from build123d import *

# Parameters (mm, degrees)
EXTRUDE_1_DEPTH     = 5
SKETCH_1_3_W        = 20
SKETCH_1_3_H        = 5
EXTRUDE_2_DEPTH     = 10
SKETCH_1_4_W        = 20
SKETCH_1_4_H        = 5
EXTRUDE_3_DEPTH     = 25
SKETCH_2_R          = 2.5
CUT_EXTRUDE_1_DEPTH = 25
CUT_EXTRUDE_2_DEPTH = 5
SKETCH_4_R          = 2.5
EXTRUDE_4_DEPTH     = 5


with BuildPart() as part:
    # 草圖1 → 填料-伸長1 (new body)
    with BuildSketch(Plane(origin=(0, 0, 0), x_dir=(1, 0, 0), z_dir=(0, 1, 0))):
        with BuildLine():
            Line((20, 10), (20, 5))
            Line((20, 5), (20, 0))
            ThreePointArc((20, 0), (23.535533906, 1.464466094), (25, 5))
            Line((25, 5), (25, 10))
            Line((25, 10), (20, 10))
        make_face()
    extrude(amount=EXTRUDE_1_DEPTH)

    # 草圖1<3> → 填料-伸長2 (add)
    with BuildSketch(Plane(origin=(0, 0, 0), x_dir=(1, 0, 0), z_dir=(0, 1, 0))):
        with Locations((10, 2.5)):
            Rectangle(SKETCH_1_3_W, SKETCH_1_3_H)
    extrude(amount=EXTRUDE_2_DEPTH)

    # 草圖1<4> → 填料-伸長3 (add)
    with BuildSketch(Plane(origin=(0, 0, 0), x_dir=(1, 0, 0), z_dir=(0, 1, 0))):
        with Locations((10, 7.5)):
            Rectangle(SKETCH_1_4_W, SKETCH_1_4_H)
    extrude(amount=EXTRUDE_3_DEPTH)

    # 草圖2 → 除料-伸長1 (cut)
    with BuildSketch(Plane.XY.offset(-5)):
        with Locations((15, 15)):
            Circle(SKETCH_2_R)
        Polygon((10, 25), (20, 20), (20, 25), align=None)
    extrude(amount=-CUT_EXTRUDE_1_DEPTH, mode=Mode.SUBTRACT)

    # 草圖3 → 除料-伸長2 (cut)
    with BuildSketch(Plane.XY):
        Polygon((20, 5), (5, 10), (20, 10), align=None)
    extrude(amount=-CUT_EXTRUDE_2_DEPTH, mode=Mode.SUBTRACT)

    # 草圖4 → 填料-伸長4 (add)
    with BuildSketch(Plane(origin=(0, 0, 0), x_dir=(0, 0, -1), z_dir=(1, 0, 0))):
        with BuildLine():
            Line((0, 10), (-10, 10))
            ThreePointArc((-10, 10), (-13.535533906, 8.535533906), (-15, 5))
            Line((-15, 5), (-15, 0))
            Line((-15, 0), (0, 0))
            Line((0, 0), (0, 10))
        make_face()
        with Locations((-10, 5)):
            Circle(SKETCH_4_R, mode=Mode.SUBTRACT)
    extrude(amount=EXTRUDE_4_DEPTH)


solid = part.part
Could you check a few things on this model? Use its own coordinates, in mm. A direction names the side the tool comes from. Give positions to 0.01 mm unless a question says otherwise; leave off trailing zeros. Order: outer loops, then holes, each group sorted by start corner. A loop starts at its lowest first (then second) coordinate and runs counter-clockwise, first axis right, second up.
1. Suppose I cut it at C-C (x = 11). List the corners of the cut face in (y, z) for me.
2. Suppose I cut it at A-A (y = 13.5). List the corners of the cut face in (x, z) for me, plus the area to 3 significant figures.
3. I need wall thicknesses on L1, parallel to Z at x = 4.5, y = 10.5; L2, parallel to Y at x = 15, z = -8.4; L3, parallel to X at y = 7.5, z = 7.75. Which ranges of each line are inside material? Lowest first, please.
4. We'd pull the mould along Z, two halves only. Please class faces 4 (the cylindrical face through (2.46, 6.69, 11.84)), 5 (the flat face through (25, 2, -7)), 6 (the flat face through (12, 4, 0)): pulls with the +Z half, pulls with the -Z half, needs draft (parallel to the pull), parting line crosses it, or undercut.
5. For faces 1 (the flat face through (12.605, 7.465, -2.465)), 2 (the flat face through (22, 5, -5)), 3 (the flat face through (5, 5, 6)), which set-ups out of +Z, -Z, +X, -X, +Y, -Y let a thin tool reach every point of the face, with its end or its side?
6. Suppose I cut it at D-D (z = -1). List the corners of the cut face in (x, y) for me, plus the area to 4 significant figures.
7. Suppose I cut it at B-B (x = 2.5). List the corners of the cut face in (y, z) for me, plus the area to 3 significant figures.
8. Will these pins go through, and if not, where does the flat tip stop? P1, Ø8, axis at y = 6, z = 5.5, coming from the +X side; P2, Ø10, axis at x = 8, y = 19, coming from the +Z side; P3, Ø4, axis at x = 2, z = 0.5, coming from the +Y side.
Solved:
1. outline: (0, -10) - (24.5, -10) - (24.5, -5) - (8, -5) - (8, 0) - (0, 0) - close
2. outline: (0, -10) - (13, -10) - (13, -5) - (0, -5) - close; (17, -10) - (20, -10) - (20, -5) - (17, -5) - close
2. area: 80.0 mm2
3. L1: z = -10 to -5
3. L2: y = 0 to 12.5, 17.5 to 22.5
3. L3: x = 0 to 5
4. face 4: undercut
4. face 5: needs draft
4. face 6: pulls with the +Z half
5. face 1: +Z, +X, +Y
5. face 2: +Z, -Z, +X, +Y
5. face 3: +Z, +X, +Y, -Y
6. outline: (0, 0) - (23, 0) - (23, 5) - (20, 5) - (5, 10) - (0, 10) - close
6. area: 177.5 mm2
7. outline: (0, -10) - (25, -10) - (25, -5) - (10, -5) - (10, 10) arc R5 ccw to (5, 15) - (0, 15) - close; hole circle Ø5 at (5, 10)
7. area: 300 mm2
8. P1: stops at x = 5
8. P2: stops at z = -5
8. P3: stops at y = 10
